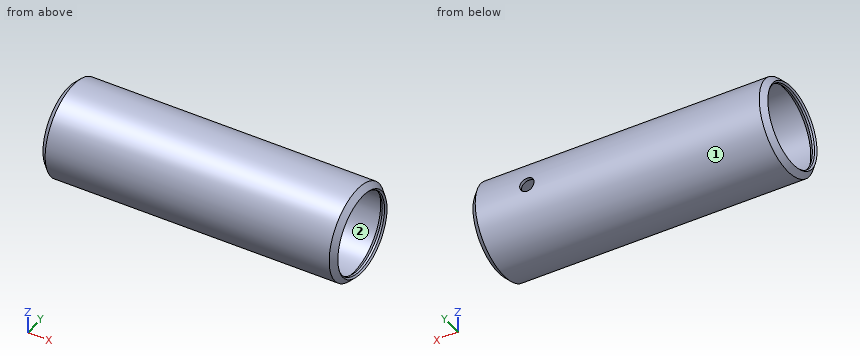
Autodesk Inventor part; units mm, degrees
ref_plane "o1_XY" through (0, -7.8105, 0) normal (1, 0, 0) x (0, 0, -1)
ref_plane "o1_YZ" through (0, -7.8105, 0) normal (0, 0, -1) x (0, 1, 0)
ref_plane "o1_ZX" through (0, -7.8105, 0) normal (0, 1, 0) x (1, 0, 0)
sketch "Sketch_5" plane through (0, 0, 0) normal (0, 0, 1) x (1, 0, 0)
  line L0 (49.2252, 0) -> (-49.2252, 0)
  line L1 (0, 6.9051) -> (0.263, 6.6421)
  line L2 (0.263, 6.6421) -> (0.635, 6.6421)
  line L3 (0.635, 6.6421) -> (1.27, 7.2771)
  line L4 (1.27, 7.2771) -> (47.9552, 7.2771)
  line L5 (47.9552, 7.2771) -> (48.5902, 6.6421)
  line L6 (48.5902, 6.6421) -> (48.9622, 6.6421)
  line L7 (48.9622, 6.6421) -> (49.2252, 6.9051)
  line L8 (49.2252, 6.9051) -> (48.3198, 7.8105)
  line L9 (48.3198, 7.8105) -> (0.9054, 7.8105)
  line L10 (0.9054, 7.8105) -> (0, 6.9051)
revolve "Revolution1" add sketch "Sketch_5" angle 360 about axis through (49.2252, 0, 0) along (1, 0, 0)
sketch "Sketch_1" plane through (0, 0, 0) normal (0, 0, 1) x (1, 0, 0)
  line L0 (39.7002, 0) -> (39.7002, 7.8105)
  line L1 (39.7002, 7.8105) -> (40.894, 7.8105)
  line L2 (40.894, 7.8105) -> (40.894, 0)
  line L3 (40.894, 0) -> (39.7002, 0)
  line L4 (39.7002, 0) -> (39.7002, 7.8105)
revolve "Revolution2" cut sketch "Sketch_1" angle 360 about axis through (39.7002, 0, 0) along (0, -1, 0)
ref_plane "o1_XY" through (0, -7.8105, 0) normal (1, 0, 0) x (0, 0, -1)
ref_plane "o1_YZ" through (0, -7.8105, 0) normal (0, 0, -1) x (0, 1, 0)
ref_plane "o1_ZX" through (0, -7.8105, 0) normal (0, 1, 0) x (1, 0, 0)
ref_plane "o2_XY" through (0, 7.8105, 0) normal (1, 0, 0) x (0, 0, -1)
ref_plane "o2_YZ" through (0, 7.8105, 0) normal (0, 0, -1) x (0, 1, 0)
ref_plane "o2_ZX" through (0, 7.8105, 0) normal (0, 1, 0) x (1, 0, 0)
ref_plane "t1_XY" through (24.6126, 7.8105, 0) normal (1, 0, 0) x (0, 0, -1)
ref_plane "t1_YZ" through (24.6126, 7.8105, 0) normal (0, 0, -1) x (0, 1, 0)
ref_plane "t1_ZX" through (24.6126, 7.8105, 0) normal (0, 1, 0) x (1, 0, 0)
ref_plane "t2_XY" through (24.6126, 0, -7.8105) normal (1, 0, 0) x (0, 0, -1)
ref_plane "t2_YZ" through (24.6126, 0, -7.8105) normal (0, 0, -1) x (0, 1, 0)
ref_plane "t2_ZX" through (24.6126, 0, -7.8105) normal (0, 1, 0) x (1, 0, 0)
ref_plane "t3_XY" through (24.6126, -7.8105, 0) normal (1, 0, 0) x (0, 0, -1)
ref_plane "t3_YZ" through (24.6126, -7.8105, 0) normal (0, 0, -1) x (0, 1, 0)
ref_plane "t3_ZX" through (24.6126, -7.8105, 0) normal (0, 1, 0) x (1, 0, 0)
ref_plane "t4_XY" through (24.6126, 0, 7.8105) normal (1, 0, 0) x (0, 0, -1)
ref_plane "t4_YZ" through (24.6126, 0, 7.8105) normal (0, 0, -1) x (0, 1, 0)
ref_plane "t4_ZX" through (24.6126, 0, 7.8105) normal (0, 1, 0) x (1, 0, 0)
ref_plane "tube1_XY" through (1.27, 0, 0) normal (1, 0, 0) x (0, 0, -1)
ref_plane "tube1_YZ" through (1.27, 0, 0) normal (0, 0, -1) x (0, 1, 0)
ref_plane "tube1_ZX" through (1.27, 0, 0) normal (0, 1, 0) x (1, 0, 0)
ref_plane "tube2_XY" through (47.9552, 0, 0) normal (1, 0, 0) x (0, 0, -1)
ref_plane "tube2_YZ" through (47.9552, 0, 0) normal (0, 0, -1) x (0, 1, 0)
ref_plane "tube2_ZX" through (47.9552, 0, 0) normal (0, 1, 0) x (1, 0, 0)
properties part number "D-75938XP-1.938"
Source: CAD feature listing. Evaluate the final solid. Frame: model axes, mm. Face numbers are marked on the shaded views. A direction names the side the tool comes from. Give positions to 0.01 mm unless a question says otherwise; leave off trailing zeros. Loops run counter-clockwise (first coordinate to the right, second up) from the corner with the lowest first, then second, coordinate; pieces in that order, holes last. Notation, with made-up numbers: (78, 75.5) -> (94, 75.5) arc R8 cw to (94, 85.5) -> close; hole circle Ø10 at (88.5, -12). An arc over 180 degrees is marked (long way). Put each result on its own line as item: value. Start each with the question number.
1) Cut plane C-C (x = 16). Return loops of the section in (y, z), then the cut area to 3 significant figures.
2) Reachability of the marked faces 1 and 2 from +Z, -Z, +X, -X, +Y, -Y: full face, straight path, thin tool, end or side. Return the list, or none.
3) Contact query for flat-ended pins moving along their axis: P1, Ø6, axis at x = 40.5, z = -1, coming from the +Y side; P2, Ø5, axis at x = 35, z = 4, coming from the -Y side; P3, Ø1, axis at x = 37.5, z = -3.5, coming from the -Y side; P4, Ø8, axis at y = 0, z = 0, coming from the +X side. Output: stop coordinate, or through.
4) Material intervals for probe 1 along Z at (x, y) = (34, 0.25); probe 2 along Z at (x, y) = (37, 1); probe 3 along Y at (x, z) = (17, 1.5), sorted ascending.
5) Cut plane A-A (z = 0). State how many separate pieces and enclosed holes the cut face has, then the cut area to 3 significant figures.
Results are:
1. outline: circle Ø15.62 at (0, 0); hole circle Ø14.55 at (0, 0)
1. area: 25.3 mm2
2. face 1: +X, -X
2. face 2: none
3. P1: stops at y = 7.81
3. P2: stops at y = -7.67
3. P3: stops at y = -7.21
3. P4: passes through
4. probe 1: z = -7.81 to -7.27, 7.27 to 7.81
4. probe 2: z = -7.75 to -7.21, 7.21 to 7.75
4. probe 3: y = -7.67 to -7.12, 7.12 to 7.67
5. separate pieces: 3
5. enclosed holes: 0
5. area: 51.9 mm2
